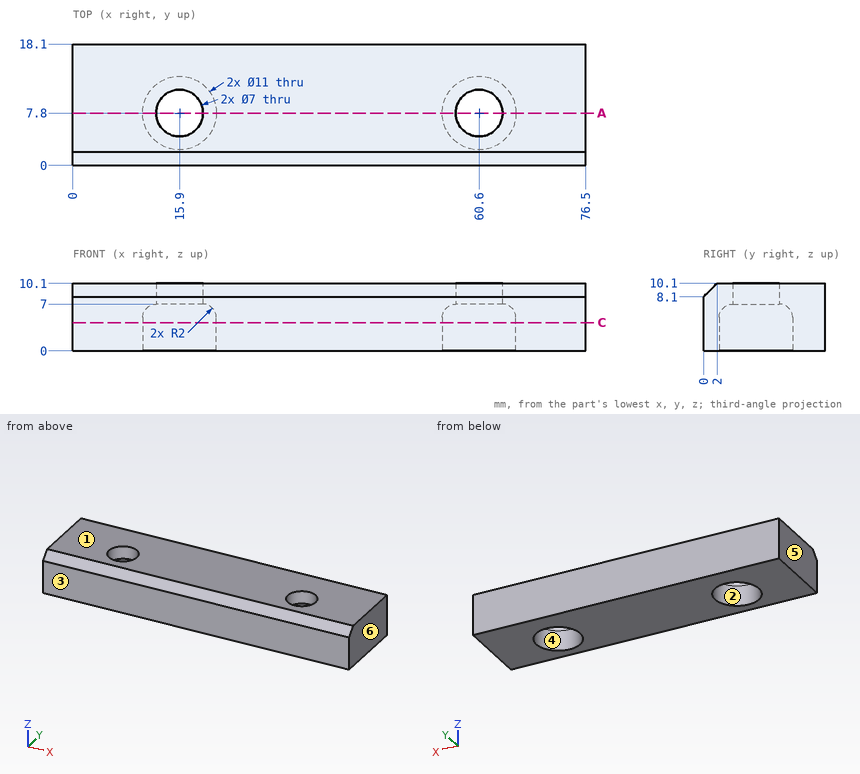
Can you work these out from the drawing? Everything is in mm from the part's minimum corner. A direction names the side the tool comes from. Give positions to 0.01 mm unless a question says otherwise; leave off trailing zeros. Order: outer loops, then holes, each group sorted by start corner. A loop starts at its lowest first (then second) coordinate and runs counter-clockwise, first axis right, second up. Notation, with made-up numbers: M -32.75,-14.75 L 6.25,-14.75 A23 ccw 6.25,22.25 Z; hole C -20,13 d5. An arc over 180 degrees is marked long. Use a Markdown table: item, result. Add a question column.
Item 1: If I drill on L1, parallel to X at y = 8, z = 3; L2, parallel to Y at x = 16, z = 1.5; L3, parallel to X at y = 9.75, z = 2.75, over which ranges is the centre line in solid material (lowest first)? Write a range as [from, to].
Item 2: Will these pins go through, and if not, where does the flat tip stop? pin 1 (7.5 mm diameter, centred on x = 15, y = 7.5, fed in from -Z); pin 2 (5.5 mm diameter, centred on x = 62, y = 9.5, fed in from -Z).
Item 3: For the marked faces 1 and 2, which set-ups out of +Z, -Z, +X, -X, +Y, -Y let a thin tool reach every point of the face, with its end or its side?
Item 4: Suppose I cut it at C-C (z = 4.25). List the corners of the cut face in (x, y) for me, then the cut area to 3 significant figures.
Item 5: Suppose I cut it at A-A (y = 7.8). Count the separate pieces of the cut face and the enclosed holes in it, then the cut area to 3 significant figures.
Item 6: We'd pull the mould along X, two halves only. Please class the marked faces 3, 4, 5 and 6: +X half, -X half, draft (parallel to the pull), parting line (faces both ways), or undercut.
Answer sheet:
| question | item | result |
|---|---|---|
| 1 | L1 | x = [0, 10.4], [21.4, 55.1], [66.1, 76.5] |
| 1 | L2 | y = [0, 2.3], [13.3, 18.1] |
| 1 | L3 | x = [0, 10.76], [21.04, 55.46], [65.74, 76.5] |
| 2 | pin 1 | stops at z = 6.6 |
| 2 | pin 2 | stops at z = 6.38 |
| 3 | face 1 | +Z, +X, -X, +Y, -Y |
| 3 | face 2 | -Z |
| 4 | outline | M 0,0 L 76.5,0 L 76.5,18.1 L 0,18.1 Z; hole C 15.9,7.8 d11; hole C 60.6,7.8 d11 |
| 4 | area | 1,190 mm² |
| 5 | separate pieces | 3 |
| 5 | enclosed holes | 0 |
| 5 | area | 579 mm² |
| 6 | face 3 | draft |
| 6 | face 4 | undercut |
| 6 | face 5 | -X half |
| 6 | face 6 | +X half |
